The listing builds one solid part. Answer for the finished solid, in the listing's coordinates (mm). Face numbers are marked on the shaded views. Round coordinates to 2 decimals unless told otherwise and drop trailing zeros. Order: outer loops, then holes, each group sorted by start corner. A loop starts at its lowest first (then second) coordinate and runs counter-clockwise, first axis right, second up. Notation, with made-up numbers: (-8.5, 18.5) -> (13.5, 18.5) arc R36 cw to (13.5, 56.5) -> close; hole circle Ø1 at (3, -6). An arc over 180 degrees is marked (long way). Answer in a Markdown table with one row per item. Add a question column.
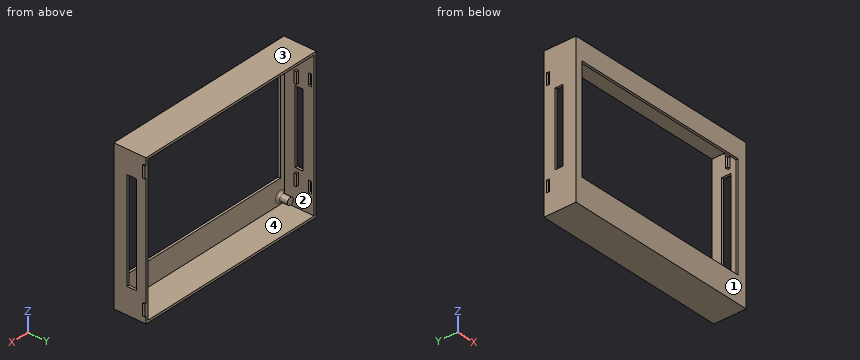
Autodesk Fusion 360 part; units mm, degrees
sketch "Sketch1" plane through (0, 0, 0) normal (0, 1, 0) x (1, 0, 0)
  line L0 (0, -130) -> (171, -130)
  line L1 (171, -130) -> (171, 0)
  line L2 (171, 0) -> (0, 0)
  line L3 (0, 0) -> (0, -130)
  line L4 (6, -113.5) -> (163, -113.5)
  line L5 (163, -113.5) -> (163, -22.5)
  line L6 (163, -22.5) -> (6, -22.5)
  line L7 (6, -22.5) -> (6, -113.5)
  line L8 (2, -128) -> (169, -128)
  line L9 (169, -128) -> (169, -2)
  line L10 (169, -2) -> (2, -2)
  line L11 (2, -2) -> (2, -128)
  circle A0 centre (6, -8.1) radius 3
  circle A1 centre (164, -8.1) radius 3
  circle A2 centre (6, -123) radius 3
  circle A3 centre (164, -123) radius 3
  dimension "d1" = 171
  dimension "d2" = 130
  dimension "d3" = 157
  dimension "d4" = 91
  dimension "d6" = 16.5
  dimension "d7" = 167
  dimension "d8" = 126
  dimension "d9" = 2
  dimension "d10" = 2
  dimension "d15" = 6
  dimension "d17" = 14.4
  dimension "d18" = 6
  dimension "d19" = 158
  dimension "d20" = 6
  dimension "d21" = 6
  dimension "d22" = 158
  dimension "d25" = 7
  dimension "d37" = 14.4
  dimension "d39" = 7
  dimension "d40" = 114.9
extrude "Extrude1" add sketch "Sketch1" along normal blind 28 contours L0 L1 L2 L3
extrude "Extrude2" add sketch "Sketch1" along normal blind 2 contours L8 L9 L10 L11 | A0 | A1 | A2 | A3
extrude "Extrude4" add sketch "Sketch1" along normal blind 10.7 contours A3
extrude "Extrude5" add sketch "Sketch1" along normal blind 10.7 contours A2
extrude "Extrude6" add sketch "Sketch1" along normal blind 10.7 contours A0
extrude "Extrude7" add sketch "Sketch1" along normal blind 10.7 contours A1
fillet "Fillet1" radius 2 1 edges at (161.203, 2, 121.9152)
fillet "Fillet2" radius 2 1 edges at (3.203, 2, 121.9152)
fillet "Fillet3" radius 2 1 edges at (3.203, 2, 7.0152)
fillet "Fillet4" radius 2 1 edges at (161.203, 2, 7.0152)
sketch "Right - Buttons" plane through (0, 0, 0) normal (1, 0, 0) x (0, 1, 0)
  line L0 (11.5, 97) -> (18.2, 97)
  line L1 (18.2, 97) -> (18.2, 33)
  line L2 (18.2, 33) -> (11.5, 33)
  line L3 (11.5, 33) -> (11.5, 97)
  line L4 (0, 0) -> (28, 0)
  line L5 (14.2, 110) -> (12.2, 110)
  line L6 (12.2, 110) -> (12.2, 100)
  line L7 (12.2, 100) -> (14.2, 100)
  line L8 (14.2, 100) -> (14.2, 110)
  line L9 (0, 130) -> (28, 130)
  line L10 (14.2, 30) -> (12.2, 30)
  line L11 (12.2, 30) -> (12.2, 20)
  line L12 (12.2, 20) -> (14.2, 20)
  line L13 (14.2, 20) -> (14.2, 30)
  line L14 (23, 112) -> (25.5, 112)
  line L15 (25.5, 112) -> (25.5, 102)
  line L16 (25.5, 102) -> (23, 102)
  line L17 (23, 102) -> (23, 112)
  line L18 (28, 0) -> (28, 130)
  line L19 (23, 28) -> (25.5, 28)
  line L20 (25.5, 28) -> (25.5, 18)
  line L21 (25.5, 18) -> (23, 18)
  line L22 (23, 18) -> (23, 28)
  dimension "d49" = 6.7
  dimension "d50" = 64
  dimension "d51" = 33
  dimension "d52" = 11.5
  dimension "d73" = 2
  dimension "d74" = 10
  dimension "d75" = 12.2
  dimension "d76" = 20
  dimension "d77" = 2
  dimension "d78" = 10
  dimension "d79" = 12.2
  dimension "d80" = 20
  dimension "d91" = 2.5
  dimension "d92" = 10
  dimension "d93" = 2.5
  dimension "d94" = 18
  dimension "d95" = 2.5
  dimension "d96" = 10
  dimension "d97" = 2.5
  dimension "d98" = 18
extrude "Extrude8" cut sketch "Right - Buttons" along normal blind 10 contours L0 L1 L2 L3
sketch "Left - HDMI" plane through (171, 0, 0) normal (1, 0, 0) x (0, 1, 0)
  line L0 (0, 130) -> (0, 0)
  line L1 (0, 0) -> (28, 0)
  line L2 (28, 0) -> (28, 130)
  line L3 (28, 130) -> (0, 130)
  line L4 (11.5, 110) -> (19.8, 110)
  line L5 (19.8, 110) -> (19.8, 22.5)
  line L6 (19.8, 22.5) -> (11.5, 22.5)
  line L7 (11.5, 22.5) -> (11.5, 110)
  line L8 (12.2, 124) -> (14.2, 124)
  line L9 (14.2, 124) -> (14.2, 114)
  line L10 (14.2, 114) -> (12.2, 114)
  line L11 (12.2, 114) -> (12.2, 124)
  line L12 (12.2, 16) -> (14.2, 16)
  line L13 (14.2, 16) -> (14.2, 6)
  line L14 (14.2, 6) -> (12.2, 6)
  line L15 (12.2, 6) -> (12.2, 16)
  line L16 (26, 124) -> (28, 124)
  line L17 (28, 124) -> (28, 114)
  line L18 (28, 114) -> (26, 114)
  line L19 (26, 114) -> (26, 124)
  line L20 (26, 16) -> (28, 16)
  line L21 (28, 16) -> (28, 6)
  line L22 (28, 6) -> (26, 6)
  line L23 (26, 6) -> (26, 16)
  dimension "d55" = 8.3
  dimension "d56" = 87.5
  dimension "d57" = 22.5
  dimension "d58" = 11.5
  dimension "d61" = 2
  dimension "d62" = 10
  dimension "d63" = 12.2
  dimension "d64" = 6
  dimension "d65" = 2
  dimension "d66" = 10
  dimension "d67" = 12.2
  dimension "d68" = 6
  dimension "d103" = 2
  dimension "d104" = 10
  dimension "d106" = 2
  dimension "d107" = 10
extrude "Extrude9" cut sketch "Left - HDMI" against normal blind 5 contours L4 L5 L6 L7
extrude "Extrude10" add sketch "Left - HDMI" against normal blind 4.5 contours L8 L9 L10 L11
extrude "Extrude11" add sketch "Left - HDMI" against normal blind 4.5 contours L12 L13 L14 L15
extrude "Extrude12" add sketch "Right - Buttons" along normal blind 4 contours L5 L6 L7 L8
extrude "Extrude13" add sketch "Right - Buttons" along normal blind 4 contours L10 L11 L12 L13
extrude "Extrude14" cut sketch "Right - Buttons" along normal blind 3 contours L14 L15 L16 L17
extrude "Extrude15" cut sketch "Right - Buttons" along normal blind 3 contours L19 L20 L21 L22
extrude "Extrude16" add sketch "Left - HDMI" along normal blind 1 contours L2 L16 L17 L18 L19
extrude "Extrude17" add sketch "Left - HDMI" along normal blind 1 contours L2 L20 L21 L22 L23
Item 1: Find the intervals of material crossed by probe 1 along X at (y, z) = (22.75, 11); probe 2 along Z at (x, y) = (74, 25.25); probe 3 along X at (y, z) = (18.5, 23.5), in increasing order. Write a range as [from, to].
Item 2: Flat-ended cylindrical pins translate along their axes: P1, Ø14, axis at y = 9.5, z = 50, coming from the +X side; P2, Ø3, axis at y = 17.5, z = 69.5, coming from the +X side; P3, Ø1.6, axis at x = 3, z = 22.5, coming from the +Y side; P4, Ø12, axis at x = 30, z = 31, coming from the +Y side. Find the tip coordinate at first contact, or state that the pin passes through.
Item 3: For a pull along Z with two mould halves and no side action, classify the marked faces 1, 2, 3 and 4 as released by +Z, released by -Z, zero draft, split by the parting line, or undercut.
Item 4: The part is cut by section B-B, the plane z = 75.5. Give the vertices of the cut face in (x, y).
Item 5: The part is cut by section C-C, the plane x = 46. Give the vertices of the cut face in (y, z), and give its area (3 significant figures).
Item 6: The part is cut by section A-A, the plane y = 8. Give the vertices of the cut face in (x, z).
Resolved:
| question | item | result |
|---|---|---|
| 1 | probe 1 | [0, 2], [169, 171] |
| 1 | probe 2 | [0, 2], [128, 130] |
| 1 | probe 3 | [0, 2] |
| 2 | P1 | x = 171 |
| 2 | P2 | x = 2 |
| 2 | P3 | y = 14.2 |
| 2 | P4 | through |
| 3 | face 1 | zero draft |
| 3 | face 2 | undercut |
| 3 | face 3 | released by +Z |
| 3 | face 4 | undercut |
| 4 | outline | (0, 0) -> (6, 0) -> (6, 2) -> (2, 2) -> (2, 11.5) -> (0, 11.5) -> close; (0, 18.2) -> (2, 18.2) -> (2, 28) -> (0, 28) -> close; (163, 0) -> (171, 0) -> (171, 11.5) -> (169, 11.5) -> (169, 2) -> (163, 2) -> close; (169, 19.8) -> (171, 19.8) -> (171, 28) -> (169, 28) -> close |
| 5 | outline | (0, 0) -> (28, 0) -> (28, 2) -> (2, 2) -> (2, 22.5) -> (0, 22.5) -> close; (0, 113.5) -> (2, 113.5) -> (2, 128) -> (28, 128) -> (28, 130) -> (0, 130) -> close |
| 5 | area | 182 mm2 |
| 6 | outline | (0, 0) -> (171, 0) -> (171, 130) -> (0, 130) -> close; circle Ø6 at (6, 8.1); circle Ø6 at (6, 123); circle Ø6 at (164, 8.1); circle Ø6 at (164, 123); hole (2, 2) -> (169, 2) -> (169, 128) -> (2, 128) -> close |
